from build123d import *

# Parameters (mm, degrees)
SKETCH1_R           = 6.985
BOSS_EXTRUDE1_DEPTH = 5.08
SKETCH3_R           = 5.08
CUT_EXTRUDE1_DEPTH  = 3.81
SKETCH4_R           = 5.08
SKETCH4_R_2         = 4.445
BOSS_EXTRUDE4_DEPTH = 3.81
FILLET2_R           = 1.27
CUT_EXTRUDE2_START  = 2.54
SKETCH5_R           = 5.715
SKETCH5_R_2         = 4.445
CUT_EXTRUDE2_DEPTH  = 2.54


with BuildPart() as part:
    # Sketch1 → Boss-Extrude1 (new body)
    with BuildSketch(Plane(origin=(0, 0, 0), x_dir=(1, 0, 0), z_dir=(0, 1, 0))):
        with Locations(Location((0, 0, 0), (0, 0, 270))):
            Circle(SKETCH1_R)
    extrude(amount=BOSS_EXTRUDE1_DEPTH)

    # Sketch3 → Cut-Extrude1 (cut)
    with BuildSketch(Plane(origin=(0, 5.08, 0), x_dir=(1, 0, 0), z_dir=(0, 1, 0))):
        with Locations(Location((0, 0, 0), (0, 0, 270))):
            Circle(SKETCH3_R)
    extrude(amount=-CUT_EXTRUDE1_DEPTH, mode=Mode.SUBTRACT)

    # Sketch4 → Boss-Extrude4 (add)
    with BuildSketch(Plane(origin=(0, 5.08, 0), x_dir=(1, 0, 0), z_dir=(0, 1, 0))):
        Circle(SKETCH4_R)
        with Locations(Location((0, 0, 0), (0, 0, 270))):
            Circle(SKETCH4_R_2, mode=Mode.SUBTRACT)
    extrude(amount=-BOSS_EXTRUDE4_DEPTH)

    # Fillet2
    fillet2_edges = [part.edges().sort_by_distance(p)[0] for p in [
        (0, 5.08, -4.445),
    ]]
    fillet(fillet2_edges, radius=FILLET2_R)

    # Sketch5 → Cut-Extrude2 (cut)
    with BuildSketch(Plane(origin=(0, 1.27, 0), x_dir=(1, 0, 0), z_dir=(0, 1, 0)).offset(CUT_EXTRUDE2_START)):
        with Locations(Location((0, 0, 0), (0, 0, 270))):
            Circle(SKETCH5_R)
        Circle(SKETCH5_R_2, mode=Mode.SUBTRACT)
    extrude(amount=-CUT_EXTRUDE2_DEPTH, mode=Mode.SUBTRACT)


solid = part.part
Input: part model. Units: mm. Frame: model coordinates. A direction names the side the tool comes from. Coordinates: 2 decimals unless noted, no trailing zeros. Write each loop counter-clockwise with the first axis right and the second up, starting at its lowest first coordinate (ties: lowest second). Pieces come first, ordered by that corner, then holes. Notation, with made-up numbers: M -26.5,53.25 L -19.5,53.25 A20 cw -19.5,68.25 Z; hole C 66,80.5 d10. An arc over 180 degrees is marked long. Answer as a JSON object with one key per item and string values. Group by question number.
(1) Set-up query: faces 1 (the face through (0, 1.27, 0)), 2 (the face through (0, 0, 0)). Return all of +Z, -Z, +X, -X, +Y, -Y with unobstructed straight access to the full face (end or side cutting, diameter ignored); none if empty.
(2) Section C-C on z = 0. Output: boundary loops of the cut face in (x, y) (3 decimals), plus the area to 3 significant figures.
(3) Ray query, line 1 along Y through (x, z) = (-1.25, -5.5); line 2 along X through (y, z) = (2.7, 0) (3 decimals); line 3 along Y through (x, z) = (1, 3.75). Return the intervals inside material, ascending. Write a range as [from, to].
(4) Mould query, pull axis X, two halves, no side actions, for faces 3 (the face through (-5, 3.81, 0)), 4 (the face through (6.926, 2.504, -0.909)), 5 (the face through (-6, 5.08, 0)). Classes: pulls with the +X half, pulls with the -X half, needs draft (parallel to the pull), parting line crosses it, or undercut.
(5) Section D-D on y = 4.55. Output: boundary loops of the cut face in (x, z) (3 decimals), plus the area to 3 significant figures.
(6) Contact query for flat-ended pins moving along their axis: P1, Ø1.5, axis at x = 4.5, y = 4.5, coming from the +Z side; P2, Ø3, axis at y = 3, z = -5, coming from the -X side; P3, Ø3, axis at x = -3.5, y = 3, coming from the -Z side. Output: stop coordinate, or through.
(7) Section A-A on y = 1.45. Output: boundary loops of the cut face in (x, z) (3 decimals), plus the area to 3 significant figures.
(8) Section B-B on x = 0. Output: boundary loops of the cut face in (y, z) (3 decimals), plus the area to 3 significant figures.
Result set:
{
 "1": {"face 1": "none", "face 2": "+Z, -Z, +X, -X, -Y"},
 "2": {"outline": "M -6.985,0 L 6.985,0 L 6.985,5.08 L 5.715,5.08 A1.27 ccw 4.445,3.81 L 5.715,3.81 L 5.715,1.27 L -5.715,1.27 L -5.715,3.81 L -4.445,3.81 A1.27 ccw -5.715,5.08 L -6.985,5.08 Z", "area": "30.0 mm2"},
 "3": {"line 1": "y = [0, 1.27], [3.81, 5.08]", "line 2": "x = [-6.985, -5.715], [5.715, 6.985]", "line 3": "y = [0, 1.27]"},
 "4": {"face 3": "undercut", "face 4": "parting line crosses it", "face 5": "needs draft"},
 "5": {"outline": "C 0,0 d13.97; hole C 0,0 d9.366", "area": "84.4 mm2"},
 "6": {"P1": "stops at z = 5.89", "P2": "stops at x = -6.04", "P3": "stops at z = -6.69"},
 "7": {"outline": "C 0,0 d13.97; hole C 0,0 d11.43", "area": "50.7 mm2"},
 "8": {"outline": "M 0,-6.985 L 5.08,-6.985 L 5.08,-5.715 A1.27 ccw 3.81,-4.445 L 3.81,-5.715 L 1.27,-5.715 L 1.27,5.715 L 3.81,5.715 L 3.81,4.445 A1.27 ccw 5.08,5.715 L 5.08,6.985 L 0,6.985 Z", "area": "30.0 mm2"}
}
